Geometry: final body of the model. Coordinates: model frame, mm. A direction names the side the tool comes from. Round coordinates to 2 decimals unless told otherwise and drop trailing zeros. Order: outer loops, then holes, each group sorted by start corner. A loop starts at its lowest first (then second) coordinate and runs counter-clockwise, first axis right, second up. Notation, with made-up numbers: M 19.5,-31.75 L 32.5,-31.75 A10 cw 32.5,-14.75 Z; hole C -20,2 d6. An arc over 180 degrees is marked long. Return JSON: item names as keys, results as strings. Group by question number.
Q1. Cut plane D-D on x = 63.5. Output: boundary loops of the cut face in (y, z).
Q2. Access query for faces 1 (the face through (-67, 10.75, 12)), 2 (the face through (68, 10.75, 12)), 3 (the face through (19.1, -19.4, 25)). Directions: +Z, -Z, +X, -X, +Y, -Y. A direction counts if a zero-diameter tool reaches every point of the face in a straight line with its end or side. Return the directions, or none.
Q3. Cut plane C-C on z = 10. Output: boundary loops of the cut face in (x, y), and give its area (3 significant figures).
Q4. Mould query, pull axis X, two halves, no side actions, for faces 4 (the face through (16.453, 5.181, 54.756)), 5 (the face through (-68, -10.75, 12)), 6 (the face through (42.3, -34.86, 12.32)). Classes: released by +X, released by -X, zero draft, split by the parting line, or undercut.
Q5. Contact query for flat-ended pins moving along their axis: pin 1 (3 mm diameter, centred on x = -6, y = -18, fed in from -Z); pin 2 (1.5 mm diameter, centred on y = -24.5, z = 44.5, fed in from +X); pin 3 (7.5 mm diameter, centred on x = -64, z = 17, fed in from -Y); pin 4 (7.5 mm diameter, centred on x = -62.5, z = 17, fed in from +Y). Output: stop coordinate, or through.
Q6. Cut plane B-B on y = 0. Output: boundary loops of the cut face in (x, z), and give its area (3 significant figures).
Q7. Cut plane A-A on x = 0. Output: boundary loops of the cut face in (y, z), and give its area (3 significant figures).
Q8. Ray query, probe 1 along Z at (x, y) = (-19, 33.5); probe 2 along Y at (x, z) = (-2.5, 96.5); probe 3 along Y at (x, z) = (0, 66). Return the intervals inside material, ascending.
```python
from build123d import *

# Parameters (mm, degrees)
BOSS_EXTRUDE1_DEPTH = 25
CUT_EXTRUDE1_REACH  = 144.302
SKETCH4_R           = 17.25


with BuildPart() as part:
    # Sketch1 → Boss-Extrude1 (new body)
    with BuildSketch(Plane.XY):
        with BuildLine():
            Line((-2.5, 45), (2.5, 45))
            Line((2.5, 45), (81, 25))
            Line((81, 25), (81, 10.75))
            Line((81, 10.75), (53.75, 10.75))
            ThreePointArc((53.75, 10.75), (43, 0), (53.75, -10.75))
            Line((53.75, -10.75), (81, -10.75))
            Line((81, -10.75), (81, -25))
            Line((81, -25), (2.5, -45))
            Line((2.5, -45), (-2.5, -45))
            Line((-2.5, -45), (-81, -25))
            Line((-81, -25), (-81, -10.75))
            Line((-81, -10.75), (-53.75, -10.75))
            ThreePointArc((-53.75, -10.75), (-43, 0), (-53.75, 10.75))
            Line((-53.75, 10.75), (-81, 10.75))
            Line((-81, 10.75), (-81, 25))
            Line((-81, 25), (-2.5, 45))
        make_face()
    extrude(amount=BOSS_EXTRUDE1_DEPTH)

    # Sketch3 → Revolve1 (revolve)
    with BuildSketch(Plane(origin=(0, 0, 0), x_dir=(0, 0, -1), z_dir=(1, 0, 0)), mode=Mode.PRIVATE) as revolve1_sk:
        Polygon((-25, 26.75), (-108, 24.75), (-108, 0), (-25, 0), align=None)
    revolve(revolve1_sk.sketch.rotate(Axis((0, 0, 220.421976321), (0, 0, -1)), 90), axis=Axis((0, 0, 220.421976321), (0, 0, -1)))

    # Sketch4 → Cut-Extrude1 (cut, up to next)
    with BuildSketch(Plane.XY.offset(108), mode=Mode.PRIVATE) as cut_extrude1_sk1:
        Circle(SKETCH4_R)
    cut_extrude1_tool1 = extrude(cut_extrude1_sk1.sketch, amount=-CUT_EXTRUDE1_REACH, mode=Mode.PRIVATE) & part.part
    add(cut_extrude1_tool1.solids().sort_by_distance((0, 0, 108))[0], mode=Mode.SUBTRACT)


solid = part.part
```
Result sheet:
{
 "1": {"outline": "M -29.46,0 L -10.75,0 L -10.75,25 L -29.46,25 Z; M 10.75,0 L 29.46,0 L 29.46,25 L 10.75,25 Z"},
 "2": {"face 1": "+Z, -Z, -X", "face 2": "+Z, -Z, +X", "face 3": "+Z"},
 "3": {"outline": "M -81,-25 L -2.5,-45 L 2.5,-45 L 81,-25 L 81,-10.75 L 53.75,-10.75 A10.75 cw 53.75,10.75 L 81,10.75 L 81,25 L 2.5,45 L -2.5,45 L -81,25 L -81,10.75 L -53.75,10.75 A10.75 cw -53.75,-10.75 L -81,-10.75 Z; hole C 0,0 d34.5", "area": "8,970 mm²"},
 "4": {"face 4": "undercut", "face 5": "zero draft", "face 6": "released by +X"},
 "5": {"pin 1": "stops at z = 0", "pin 2": "stops at x = 11.25", "pin 3": "stops at y = -30.29", "pin 4": "stops at y = 30.67"},
 "6": {"outline": "M -43,0 L -17.25,0 L -17.25,108 L -24.75,108 L -26.75,25 L -43,25 Z; M 17.25,0 L 43,0 L 43,25 L 26.75,25 L 24.75,108 L 17.25,108 Z", "area": "2,700 mm²"},
 "7": {"outline": "M -45,0 L -17.25,0 L -17.25,108 L -24.75,108 L -26.75,25 L -45,25 Z; M 17.25,0 L 45,0 L 45,25 L 26.75,25 L 24.75,108 L 17.25,108 Z", "area": "2,800 mm²"},
 "8": {"probe 1": "z = 0 to 25", "probe 2": "y = -24.9 to -17.07, 17.07 to 24.9", "probe 3": "y = -25.76 to -17.25, 17.25 to 25.76"}
}
